The figure shows three views and two pictorial views of one solid part (mm, origin at its lowest corner). Answer the questions. Give positions to 0.01 mm unless a question says otherwise; leave off trailing zeros. Loops run counter-clockwise (first coordinate to the right, second up) from the corner with the lowest first, then second, coordinate; pieces in that order, holes last. Notation, with made-up numbers: (6.5, 15.25) - (36.5, 15.25) arc R34 ccw to (36.5, 50.25) - close; hole circle Ø10 at (47, 58). An arc over 180 degrees is marked (long way). Use a Markdown table: item, result. Add a question column.
Item 1: A cutting plane is placed at C-C (x = 354). Determine the outline of the cut face in (y, z).
Item 2: A cutting plane is placed at A-A (y = 331.5). Determine the outline of the cut face in (x, z).
Item 3: Consider probe 1 along X at (y, z) = (137.5, 4.5); probe 2 along X at (y, z) = (348.5, 7) (1 decimal); probe 3 along Y at (x, z) = (737, 1.25). Determine where each line is inside the solid, lowest interval first. Write a range as [from, to].
Item 4: Each of these flat-tipped pins is pushed along its axis until it touches: P1, Ø4, axis at x = 662, z = 3, coming from the +Y side; P2, Ø1, axis at x = 521, z = 3.5, coming from the +Y side. Where does it stop, or does it pass through?
Item 5: A cutting plane is placed at D-D (x = 561.5). Determine the outline of the cut face in (y, z) (1 decimal).
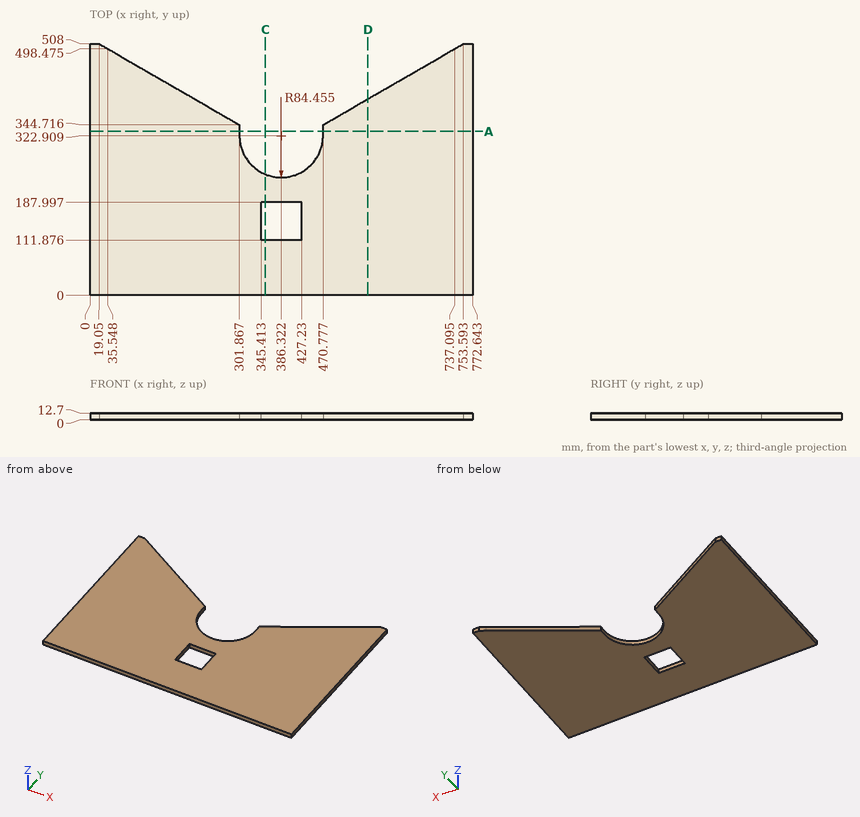
Geometry says:
| question | item | result |
|---|---|---|
| 1 | outline | (0, 0) - (111.88, 0) - (111.88, 12.7) - (0, 12.7) - close; (188, 0) - (244.88, 0) - (244.88, 12.7) - (188, 12.7) - close |
| 2 | outline | (0, 0) - (301.87, 0) - (301.87, 12.7) - (0, 12.7) - close; (470.78, 0) - (772.64, 0) - (772.64, 12.7) - (470.78, 12.7) - close |
| 3 | probe 1 | [0, 345.41], [427.23, 772.64] |
| 3 | probe 2 | [0, 295.3], [477.3, 772.6] |
| 3 | probe 3 | [0, 498.42] |
| 4 | P1 | y = 456.27 |
| 4 | P2 | y = 374 |
| 5 | outline | (0, 0) - (397.1, 0) - (397.1, 12.7) - (0, 12.7) - close |
